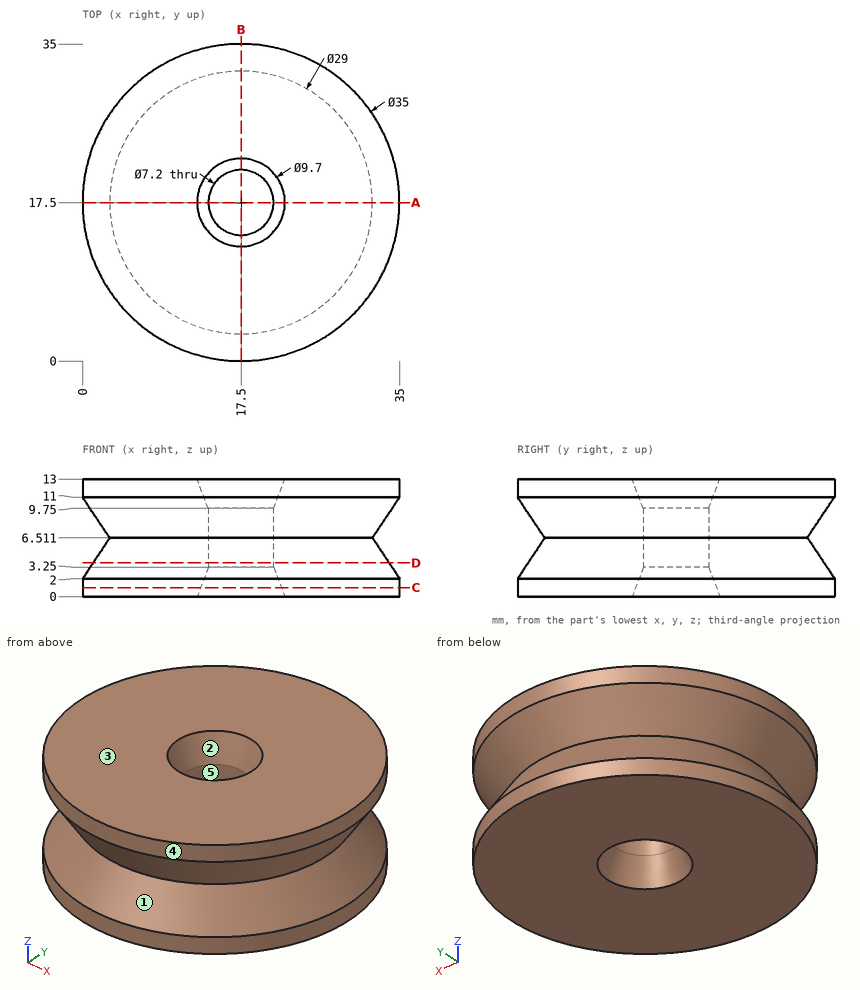
Input: dimensioned drawing with shaded views. Units: mm. Origin: part minimum x, y, z. A direction names the side the tool comes from. Round coordinates to 2 decimals unless told otherwise and drop trailing zeros. Order: outer loops, then holes, each group sorted by start corner. A loop starts at its lowest first (then second) coordinate and runs counter-clockwise, first axis right, second up. Notation, with made-up numbers: (-18.5, -20.5) - (-4.5, -20.5) arc R27 cw to (-4.5, 14.5) - close; hole circle Ø11 at (19, 34.25). An arc over 180 degrees is marked (long way). Write item = value, one per line. Start each with the question number.
Q1. Pin query (flat end, axial travel): pin 1 (6 mm diameter, centred on x = 24, z = 5, fed in from -Y); pin 2 (10 mm diameter, centred on x = 19.5, y = 15, fed in from +Z); pin 3 (5 mm diameter, centred on y = 25.5, z = 8, fed in from -X); pin 4 (2 mm diameter, centred on y = 25.5, z = 3, fed in from +X) (1 decimal). Return the tip coordinate at first contact, or that it passes through.
Q2. Access query for the marked faces 1 and 2. Directions: +Z, -Z, +X, -X, +Y, -Y. A direction counts if a zero-diameter tool reaches every point of the face in a straight line with its end or side. Return the directions, or none.
Q3. Cut plane A-A on y = 17.5. Return the cut outline in (x, z), and give its area (3 significant figures).
Q4. Cut plane D-D on z = 3.75. Return the cut outline in (x, y), and give its area (3 significant figures).
Q5. Pull-direction query (X, two-part tool) for the marked faces 3, 4 and 5; classes: +X half, -X half, draft (parallel to the pull), parting line (faces both ways), or undercut.
Q6. Cut plane C-C on z = 1. Return the cut outline in (x, y) (1 decimal).
Q7. Ray query, line 1 (Y direction, x = 17.5, z = 5.5); line 2 (Y direction, x = 14.5, z = 5.5) (1 decimal); line 3 (Z direction, x = 33.5, y = 18.5) (1 decimal). Return the intervals inside material, ascending. Write a range as from..to.
Outcome:
q1.pin_1 = 1
q1.pin_2 = 13
q1.pin_3 = 1.96
q1.pin_4 = 33.2
q2.face_1 = none
q2.face_2 = +Z
q3.outline = (0, 0) - (12.65, 0) - (13.9, 3.25) - (13.9, 9.75) - (12.65, 13) - (0, 13) - (0, 11) - (3, 6.51) - (0, 2) - close; (21.1, 3.25) - (22.35, 0) - (35, 0) - (35, 2) - (32, 6.51) - (35, 11) - (35, 13) - (22.35, 13) - (21.1, 9.75) - close
q3.area = 326 mm^2
q4.outline = circle Ø32.67 at (17.5, 17.5); hole circle Ø7.2 at (17.5, 17.5)
q4.area = 798 mm^2
q5.face_3 = draft
q5.face_4 = parting line
q5.face_5 = undercut
q6.outline = circle Ø35 at (17.5, 17.5); hole circle Ø8.9 at (17.5, 17.5)
q7.line_1 = 2.33..13.9, 21.1..32.67
q7.line_2 = 2.6..15.5, 19.5..32.4
q7.line_3 = 0..4.2, 8.8..13
